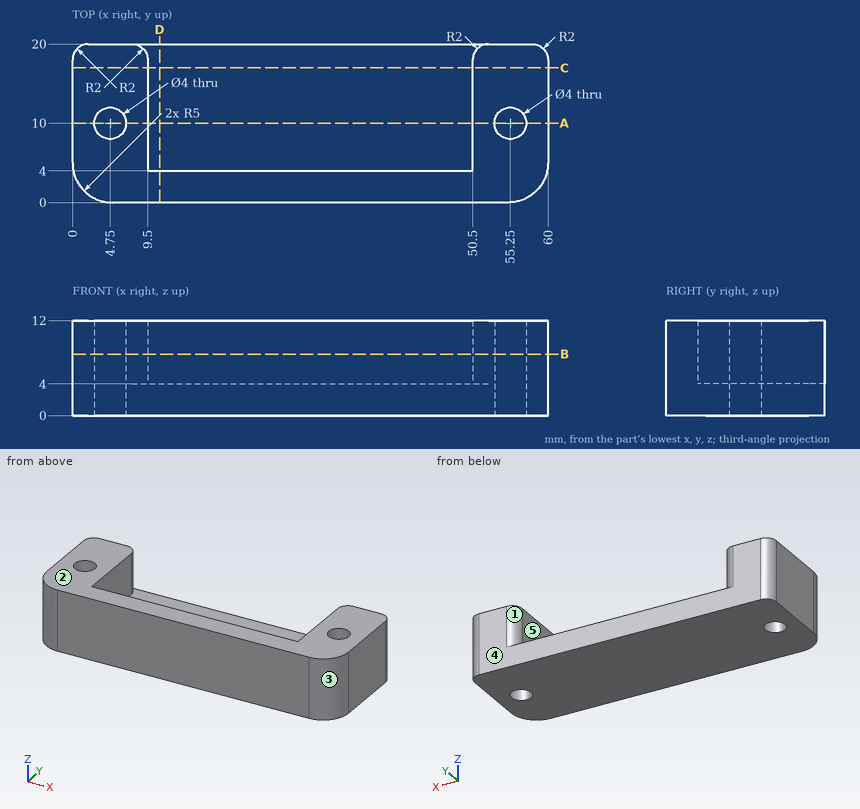
Could you check a few things on this drawing? It's one solid part, dimensions in mm from its lowest x, y, z. A direction names the side the tool comes from. Coordinates: 2 decimals unless noted, no trailing zeros. Write each loop counter-clockwise with the first axis right and the second up, starting at its lowest first coordinate (ties: lowest second). Pieces come first, ordered by that corner, then holes.
1) If I drill on line 1 (X direction, y = 10, z = 3.5); line 2 (X direction, y = 10, z = 7); line 3 (X direction, y = 17.75, z = 11.75), over which ranges is the centre line in solid material (lowest first)?
Filled in:
line 1: x = 0 to 2.75, 6.75 to 53.25, 57.25 to 60
line 2: x = 0 to 2.75, 6.75 to 9.5, 50.5 to 53.25, 57.25 to 60
line 3: x = 0 to 9.5, 50.5 to 60
2) I'm going to push flat-ended pins straight in: pin 1 (6 mm diameter, centred on x = 38.5, y = 12.5, fed in from +Z); pin 2 (4 mm diameter, centred on x = 39, z = 6.5, fed in from +Y). Where does each tip first touch, or does it pass through?
Filled in:
pin 1: stops at z = 4
pin 2: stops at y = 4
3) If we section it at B-B (z = 7.75): List the corners of the cut face in (x, y) for me.
Filled in:
outline: (0, 5) arc R5 ccw to (5, 0) - (55, 0) arc R5 ccw to (60, 5) - (60, 18) arc R2 ccw to (58, 20) - (52.5, 20) arc R2 ccw to (50.5, 18) - (50.5, 4) - (9.5, 4) - (9.5, 18) arc R2 ccw to (7.5, 20) - (2, 20) arc R2 ccw to (0, 18) - close; hole circle Ø4 at (4.75, 10); hole circle Ø4 at (55.25, 10)
4) Which directions (+Z, -Z, +X, -X, +Y, -Y) give clear straight access to the entire face, cutting with the end or side of a thin tool? Please do the marked faces 4 and 5.
Filled in:
face 4: +Z, -Z, +X, -X, +Y
face 5: +Z, +Y
5) If we section it at C-C (y = 17): List the corners of the cut face in (x, z) for me.
Filled in:
outline: (0, 0) - (60, 0) - (60, 12) - (50.5, 12) - (50.5, 4) - (9.5, 4) - (9.5, 12) - (0, 12) - close
6) If we section it at D-D (x = 11): List the corners of the cut face in (y, z) for me, plus the area to 3 significant figures.
Filled in:
outline: (0, 0) - (20, 0) - (20, 4) - (4, 4) - (4, 12) - (0, 12) - close
area: 112 mm2
7) Thinking about a two-plate mould opening in X: for the marked faces 1, 2 and 3, which applies, +X half, -X half, draft (parallel to the pull), parting line (faces both ways), or undercut?
Filled in:
face 1: undercut
face 2: draft
face 3: +X half
8) If we section it at A-A (y = 10): List the corners of the cut face in (x, z) for me.
Filled in:
outline: (0, 0) - (2.75, 0) - (2.75, 12) - (0, 12) - close; (6.75, 0) - (53.25, 0) - (53.25, 12) - (50.5, 12) - (50.5, 4) - (9.5, 4) - (9.5, 12) - (6.75, 12) - close; (57.25, 0) - (60, 0) - (60, 12) - (57.25, 12) - close
